Verification items for this drawing (mm, ordinates from the low corner). A direction names the side the tool comes from. Give positions to 0.01 mm unless a question says otherwise; leave off trailing zeros. Loops run counter-clockwise (first coordinate to the right, second up) from the corner with the lowest first, then second, coordinate; pieces in that order, holes last. Notation, with made-up numbers: M -4,75 L 12,75 A17 ccw 12,89 Z; hole C -15,-14.5 d9. An arc over 180 degrees is marked long. Use a Markdown table: item, result.
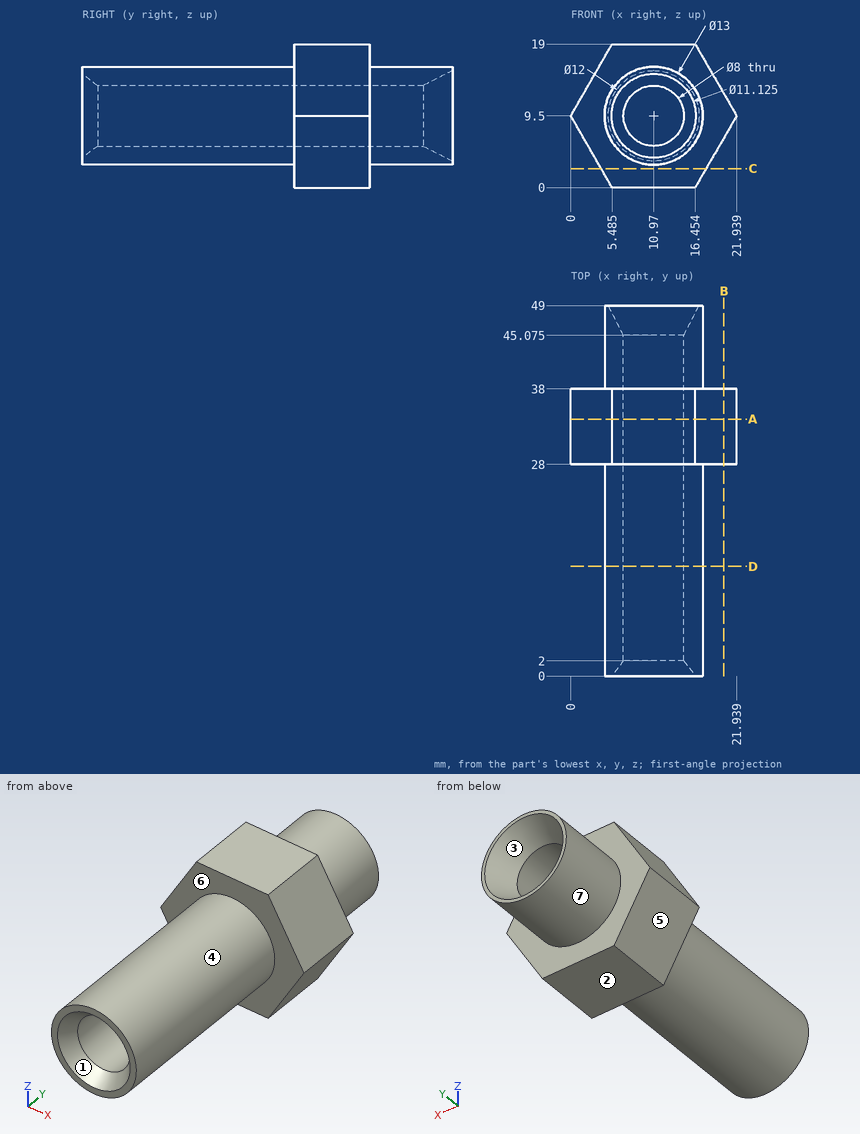
(1) Draft check along Z on the marked faces 1, 2, 3 and 4. Enter one of: +Z half, -Z half, draft (parallel to the pull), parting line (faces both ways), or undercut.
Results below:
| item | result |
|---|---|
| face 1 | undercut |
| face 2 | -Z half |
| face 3 | undercut |
| face 4 | parting line |
(2) Material ranges on line 1 (Z direction, x = 11.25, y = 6.5) (1 decimal); line 2 (X direction, y = 28.5, z = 9.5); line 3 (X direction, y = 27.5, z = 9.5), recorded low to high.
Results below:
| item | result |
|---|---|
| line 1 | 3 to 5.5, 13.5 to 16 |
| line 2 | 0 to 6.97, 14.97 to 21.94 |
| line 3 | 4.47 to 6.97, 14.97 to 17.47 |
(3) Set-up check for the marked faces 5, 6 and 7: record each of +Z, -Z, +X, -X, +Y, -Y from which the full face is reachable in a straight line by a thin tool's end or side.
Results below:
| item | result |
|---|---|
| face 5 | -Z, -X, +Y, -Y |
| face 6 | -Y |
| face 7 | +Y |
(4) Gauge pin test, flat ends, axial feed: P1, Ø2, axis at x = 12, z = 7, coming from the +Y side; P2, Ø3, axis at x = 13, y = 43, coming from the +Z side; P3, Ø5, axis at y = 38, z = 6, coming from the +X side; P4, Ø2, axis at x = 13.5, y = 6, coming from the -Z side. Record the tip position at first contact, or that the pin passes through.
Results below:
| item | result |
|---|---|
| P1 | through |
| P2 | z = 15.98 |
| P3 | x = 21.36 |
| P4 | z = 3.18 |
(5) Cross-section at D-D on y = 14.5. Record the cut outline in (x, z).
Results below:
| item | result |
|---|---|
| outline | C 10.97,9.5 d13; hole C 10.97,9.5 d8 |
(6) Cross-section at A-A on y = 34. Record the cut outline in (x, z) (1 decimal).
Results below:
| item | result |
|---|---|
| outline | M 0,9.5 L 5.5,0 L 16.5,0 L 21.9,9.5 L 16.5,19 L 5.5,19 Z; hole C 11,9.5 d8 |
(7) Cross-section at B-B on x = 20.25. Record the cut outline in (y, z) (1 decimal).
Results below:
| item | result |
|---|---|
| outline | M 28,6.6 L 38,6.6 L 38,12.4 L 28,12.4 Z |
(8) Cross-section at C-C on z = 2.5. Record the cut outline in (x, y).
Results below:
| item | result |
|---|---|
| outline | M 4.04,28 L 17.9,28 L 17.9,38 L 4.04,38 Z |
